```python
from build123d import *

# Parameters (mm, degrees)
CYLINDER008_R             = 1.65
CYLINDER008_DEPTH         = 10
CYLINDER007_R             = 7.25
CYLINDER007_DEPTH         = 1
CYLINDER006_R             = 6.5
CYLINDER006_DEPTH         = 32
FUSION005_PLACEMENT_ANGLE = 90
BOX003_W                  = 30
BOX003_H                  = 3
BOX003_DEPTH              = 15
CYLINDER003_R             = 3.25
CYLINDER003_DEPTH         = 10
CYLINDER002_R             = 5.5
CYLINDER002_DEPTH         = 6
CYLINDER005_R             = 3.25
CYLINDER005_DEPTH         = 10
CYLINDER004_R             = 5.5
CYLINDER004_DEPTH         = 6
BOX002_W                  = 30
BOX002_H                  = 20
BOX002_DEPTH              = 20
BOX001_W                  = 30
BOX001_H                  = 20
BOX001_DEPTH              = 20
BOX_W                     = 30
BOX_H                     = 63
BOX_DEPTH                 = 20
FILLET_R                  = 3


with BuildPart() as m4wormscrew:
    # Cylinder008 → Cylinder008 (new body)
    with BuildSketch(Plane(origin=(0, -3, 15), x_dir=(1, 0, 0), z_dir=(0, -1, 0))):
        Circle(CYLINDER008_R)
    extrude(amount=CYLINDER008_DEPTH)


with BuildPart() as cylinder007:
    # Cylinder007 → Cylinder007 (new body)
    with BuildSketch(Plane.XY):
        Circle(CYLINDER007_R)
    extrude(amount=CYLINDER007_DEPTH)


with BuildPart() as lasermoduletemplate001:
    # Cylinder006 → Cylinder006 (new body)
    with BuildSketch(Plane.XY):
        Circle(CYLINDER006_R)
    extrude(amount=CYLINDER006_DEPTH)

    # Fusion005: union Cylinder007
    add(cylinder007.part)


with BuildPart() as lasermoduletemplate001_1:
    # Fusion005 placement: moved
    add(lasermoduletemplate001.part.moved(Location((-15, 0, 10))).rotate(Axis((-15, 0, 10), (0, 1, 0)), FUSION005_PLACEMENT_ANGLE))


with BuildPart() as cube003:
    # Box003 → Box003 (new body)
    with BuildSketch(Plane(origin=(-15, -1.5, 15), x_dir=(1, 0, 0), z_dir=(0, 0, 1))):
        with Locations((15, 1.5)):
            Rectangle(BOX003_W, BOX003_H)
    extrude(amount=BOX003_DEPTH)


with BuildPart() as cylinder003:
    # Cylinder003 → Cylinder003 (new body)
    with BuildSketch(Plane.XY):
        Circle(CYLINDER003_R)
    extrude(amount=CYLINDER003_DEPTH)


with BuildPart() as screwthrough001:
    # Cylinder002 → Cylinder002 (new body)
    with BuildSketch(Plane.XY.offset(4)):
        Circle(CYLINDER002_R)
    extrude(amount=CYLINDER002_DEPTH)

    # Fusion001: union Cylinder003
    add(cylinder003.part)


with BuildPart() as screwthrough001_1:
    # Fusion001 placement: moved
    add(screwthrough001.part.moved(Location((0, -21.5, 0))))


with BuildPart() as cylinder005:
    # Cylinder005 → Cylinder005 (new body)
    with BuildSketch(Plane.XY):
        Circle(CYLINDER005_R)
    extrude(amount=CYLINDER005_DEPTH)


with BuildPart() as fusion004:
    # Cylinder004 → Cylinder004 (new body)
    with BuildSketch(Plane.XY.offset(4)):
        Circle(CYLINDER004_R)
    extrude(amount=CYLINDER004_DEPTH)

    # Fusion002: union Cylinder005
    add(cylinder005.part)


with BuildPart() as fusion004_1:
    # Fusion002 placement: moved
    add(fusion004.part.moved(Location((0, 21.5, 0))))

    # Fusion004: union ScrewThrough001
    add(screwthrough001_1.part)


with BuildPart() as cube002:
    # Box002 → Box002 (new body)
    with BuildSketch(Plane(origin=(-15, -31.5, 10), x_dir=(1, 0, 0), z_dir=(0, 0, 1))):
        with Locations((15, 10)):
            Rectangle(BOX002_W, BOX002_H)
    extrude(amount=BOX002_DEPTH)


with BuildPart() as fusion003:
    # Box001 → Box001 (new body)
    with BuildSketch(Plane(origin=(-15, 11.5, 10), x_dir=(1, 0, 0), z_dir=(0, 0, 1))):
        with Locations((15, 10)):
            Rectangle(BOX001_W, BOX001_H)
    extrude(amount=BOX001_DEPTH)

    # Fusion003: union Cube002
    add(cube002.part)


with BuildPart() as cut004:
    # Box → Box (new body)
    with BuildSketch(Plane(origin=(-15, -31.5, 0), x_dir=(1, 0, 0), z_dir=(0, 0, 1))):
        with Locations((15, 31.5)):
            Rectangle(BOX_W, BOX_H)
    extrude(amount=BOX_DEPTH)

    # Cut: cut Fusion003
    add(fusion003.part, mode=Mode.SUBTRACT)

    # Cut001: cut Fusion004
    add(fusion004_1.part, mode=Mode.SUBTRACT)

    # Cut002: cut Cube003
    add(cube003.part, mode=Mode.SUBTRACT)

    # Cut003: cut LaserModuleTemplate001
    add(lasermoduletemplate001_1.part, mode=Mode.SUBTRACT)

    # Fillet
    fillet_edges = [cut004.edges().sort_by_distance(p)[0] for p in [
        (0, -31.5, 10),
        (0, -11.5, 10),
        (0, -11.5, 20),
        (0, 11.5, 20),
        (0, 11.5, 10),
        (0, 31.5, 10),
    ]]
    fillet(fillet_edges, radius=FILLET_R)

    # Cut004: cut M4WormScrew
    add(m4wormscrew.part, mode=Mode.SUBTRACT)


solid = cut004.part
```
The listing builds one solid part. Answer for the finished solid, in the listing's coordinates (mm). A direction names the side the tool comes from. Give positions to 0.01 mm unless a question says otherwise; leave off trailing zeros. Order: outer loops, then holes, each group sorted by start corner. A loop starts at its lowest first (then second) coordinate and runs counter-clockwise, first axis right, second up. Notation, with made-up numbers: (-34, 84) - (-21, 84) arc R24 cw to (-21, 115) - close; hole circle Ø11 at (16, 7.25). An arc over 180 degrees is marked (long way). Answer in a Markdown table with one row per item. Add a question column.
Q1. For a pull along X with two mould halves and no side action, classify faces 1 (the flat face through (15, 0, 3)), 2 (the flat face through (-0.2, -11.5, 13.2)), 3 (the cylindrical face through (-0.215, -8.135, 16.636)) as released by +X, released by -X, zero draft, split by the parting line, or undercut.
Q2. The part is cut by section A-A (y = 21.5). Determine the outline of the cut face in (x, z).
Q3. The part is cut by section B-B (z = 8.5). Determine the outline of the cut face in (x, y).
Q4. Which of the six approach directions +Z, -Z, +X, -X, +Y, -Y give full straight-line access (tool end or side, diameter ignored) to faces 4 (the cylindrical face through (-14.507, -0.298, 2.756)), 5 (the flat face through (-4, -17, 10)), 6 (the flat face through (-4, 26, 10))?
Q5. Find the intervals of material crossed by line 1 along Y through (x, z) = (0, 0.8); line 2 along X through (y, z) = (-7.25, 15); line 3 along Y through (x, z) = (-3.5, 5.25), in increasing order. Write a range as [from, to].
Q6. The part is cut by section C-C (x = 12). Determine the outline of the cut face in (y, z), then the cut area to 3 significant figures.
Q7. The part is cut by section D-D (z = 15). Determine the outline of the cut face in (x, y), then the cut area to 3 significant figures.
Q8. Given P1, Ø1.2, axis at x = 3, z = 15, coming from the -Y side; P2, Ø4.5, axis at x = -3.5, z = 14.5, coming from the +Y side; P3, Ø11.5, axis at y = 0, z = 10, coming from the +X side; P4, Ø10, axis at x = -11, z = 16, coming from the -Y side, each flat-ended and moving along its own axis, determine where each tip first touches the part or whether it passes through.
Determined:
| question | item | result |
|---|---|---|
| 1 | face 1 | released by +X |
| 1 | face 2 | zero draft |
| 1 | face 3 | undercut |
| 2 | outline | (-15, 0) - (-3.25, 0) - (-3.25, 4) - (-5.5, 4) - (-5.5, 10) - (-15, 10) - close; (3.25, 0) - (15, 0) - (15, 10) - (5.5, 10) - (5.5, 4) - (3.25, 4) - close |
| 3 | outline | (-15, -31.1) - (15, -31.1) - (15, -6.32) - (-14, -6.32) - (-14, -7.09) - (-15, -7.09) - close; (-15, 7.09) - (-14, 7.09) - (-14, 6.32) - (15, 6.32) - (15, 31.1) - (-15, 31.1) - close; hole circle Ø11 at (0, -21.5); hole circle Ø11 at (0, 21.5) |
| 4 | face 4 | -X |
| 4 | face 5 | +Z, +X, -X, -Y |
| 4 | face 6 | +Z, +X, -X, +Y |
| 5 | line 1 | y = [-31.5, -24.75], [-18.25, 18.25], [24.75, 31.5] |
| 5 | line 2 | x = [-15, -1.65], [1.65, 15] |
| 5 | line 3 | y = [-31.5, -25.74], [-17.26, -4.44], [4.44, 17.26], [25.74, 31.5] |
| 6 | outline | (-31.5, 0) - (31.5, 0) - (31.5, 7) arc R3 ccw to (28.5, 10) - (14.5, 10) arc R3 cw to (11.5, 13) - (11.5, 17) arc R3 ccw to (8.5, 20) - (1.5, 20) - (1.5, 16.32) arc R6.5 cw (long way) to (-1.5, 16.32) - (-1.5, 20) - (-8.5, 20) arc R3 ccw to (-11.5, 17) - (-11.5, 13) arc R3 cw to (-14.5, 10) - (-28.5, 10) arc R3 ccw to (-31.5, 7) - close |
| 6 | area | 713 mm² |
| 7 | outline | (-15, -11.5) - (-1.65, -11.5) - (-1.65, -4.15) - (-14, -4.15) - (-14, -5.25) - (-15, -5.25) - close; (-15, 5.25) - (-14, 5.25) - (-14, 4.15) - (15, 4.15) - (15, 11.5) - (-15, 11.5) - close; (1.65, -11.5) - (15, -11.5) - (15, -4.15) - (1.65, -4.15) - close |
| 7 | area | 414 mm² |
| 8 | P1 | stops at y = -11.5 |
| 8 | P2 | stops at y = 11.6 |
| 8 | P3 | passes through |
| 8 | P4 | stops at y = -12.26 |
